```python
from build123d import *

# Parameters (mm, degrees)
BOSS_EXTRUDE1_DEPTH   = 70
FILLET1_R             = 2
M5_TAPPED_HOLE1_D     = 4.2
M5_TAPPED_HOLE1_DEPTH = 12.5
M5_TAPPED_HOLE1_TIP   = 1.2618073


with BuildPart() as part:
    # Sketch1 → Boss-Extrude1 (new body)
    with BuildSketch(Plane.XY):
        Polygon((0, 0), (0, 14), (35.751288694, 14), (60, 0), align=None)
    extrude(amount=BOSS_EXTRUDE1_DEPTH)

    # Fillet1
    fillet1_edges = [part.edges().sort_by_distance(p)[0] for p in [
        (17.875644347, 14, 70),
        (0, 7, 70),
        (30, 0, 70),
        (0, 7, 0),
        (17.875644347, 14, 0),
        (47.875644347, 7, 0),
        (30, 0, 0),
        (0, 0, 35),
        (0, 14, 35),
        (35.751288694, 14, 35),
        (60, 0, 35),
        (47.875644347, 7, 70),
    ]]
    fillet(fillet1_edges, radius=FILLET1_R)

    # M5 Tapped Hole1
    with Locations(Plane(origin=(0, 14, 0), x_dir=(1, 0, 0), z_dir=(0, 1, 0))):
        with Locations((8, -62), (28, -62)):
            Hole(M5_TAPPED_HOLE1_D / 2, depth=M5_TAPPED_HOLE1_DEPTH)
            with Locations((0, 0, -(M5_TAPPED_HOLE1_DEPTH + M5_TAPPED_HOLE1_TIP / 2))):  # 118° drill point
                Cone(0, M5_TAPPED_HOLE1_D / 2, M5_TAPPED_HOLE1_TIP, mode=Mode.SUBTRACT)


solid = part.part
```
Geometry check sheet. Reference: the model listing, model coordinates, mm. A direction names the side the tool comes from. Coordinates: 2 decimals unless noted, no trailing zeros. Order: outer loops, then holes, each group sorted by start corner. A loop starts at its lowest first (then second) coordinate and runs counter-clockwise, first axis right, second up. Notation, with made-up numbers: (-6.75, -30.75) - (6.25, -30.75) arc R25 cw to (6.25, -16.75) - close; hole circle Ø11 at (63.5, 12). An arc over 180 degrees is marked (long way). Answer in a Markdown table with one row per item. Add a question column.
1. Gauge pin test, flat ends, axial feed: pin 1 Ø5 at (y, z) = (6.5, 55) entering from +X; pin 2 Ø1.5 at (x, z) = (41, 27) entering from +Y. Record the tip position at first contact, or that the pin passes through.
2. Material ranges on L1, parallel to Z at x = 8, y = 11.5; L2, parallel to X at y = 6.5, z = 62; L3, parallel to X at y = 8.75, z = 62, recorded low to high. Write a range as [from, to].
3. Draft check along X on faces 1 (the face through (0.57, 7.07, 0.6)), 2 (the face through (29.666, 7.663, 63.278)), 3 (the face through (26.91, 0.57, 69.4)). Enter one of: +X half, -X half, draft (parallel to the pull), parting line (faces both ways), or undercut.
4. Section check A-A (z = 32). Enter the section's corners in (x, y).
5. Access from +Z, -Z, +X, -X, +Y, -Y to the whole of each face (thin tool, end or side, straight path). Record for faces 4 (the face through (9.666, 7.663, 63.278)), 5 (the face through (0.57, 13.4, 35.46)).
6. Section check B-B (y = 4.5). Give the number of separate pieces and of enclosed holes in the cut face, plus the area to 3 significant figures.
Data:
| question | item | result |
|---|---|---|
| 1 | pin 1 | stops at x = 53.07 |
| 1 | pin 2 | stops at y = 11.4 |
| 2 | L1 | z = [0, 59.9], [64.1, 70] |
| 2 | L2 | x = [0, 5.9], [10.1, 25.9], [30.1, 48.74] |
| 2 | L3 | x = [0, 5.9], [10.1, 25.9], [30.1, 44.84] |
| 3 | face 1 | -X half |
| 3 | face 2 | undercut |
| 3 | face 3 | draft |
| 4 | outline | (0, 2) arc R2 ccw to (2, 0) - (52.54, 0) arc R2 ccw to (53.54, 3.73) - (36.22, 13.73) arc R2 ccw to (35.22, 14) - (2, 14) arc R2 ccw to (0, 12) - close |
| 5 | face 4 | +Y |
| 5 | face 5 | +Z, -Z, -X, +Y |
| 6 | separate pieces | 1 |
| 6 | enclosed holes | 2 |
| 6 | area | 3,620 mm² |
